Design review of the part built by this model. Coordinates are the model's own, in mm. A direction names the side the tool comes from. Give positions to 0.01 mm unless a question says otherwise; leave off trailing zeros. Loops run counter-clockwise (first coordinate to the right, second up) from the corner with the lowest first, then second, coordinate; pieces in that order, holes last. Notation, with made-up numbers: (60.5, -3.75) - (95.5, -3.75) arc R18 ccw to (95.5, 12.25) - close; hole circle Ø11 at (0.5, -18). An arc over 180 degrees is marked (long way). Write each question's results on one line, items separated by ' | '.
from build123d import *

# Parameters (mm, degrees)
SKETCH1_R           = 2.2
BOSS_EXTRUDE1_DEPTH = 4
FILLET1_R           = 3
SKETCH2_W           = 4.6228
SKETCH2_H           = 4.6228
BOSS_EXTRUDE2_DEPTH = 2
FILLET2_R           = 0.508
FILLET3_R           = 0.508


with BuildPart() as part:
    # Sketch1 → Boss-Extrude1 (new body)
    with BuildSketch(Plane(origin=(0, 0, 0), x_dir=(0, 0, -1), z_dir=(1, 0, 0))):
        Polygon((-4.5, 4.5), (-17.2, 4.5), (-17.2, -4.5), (29.9, -4.5), (29.9, 4.5), (4.5, 43.87), (-4.5, 43.87), align=None)
        with Locations((25.4, 0)):
            Circle(SKETCH1_R, mode=Mode.SUBTRACT)
        with Locations((0, 13.97)):
            Circle(SKETCH1_R, mode=Mode.SUBTRACT)
        with Locations((0, 39.37)):
            Circle(SKETCH1_R, mode=Mode.SUBTRACT)
        with Locations((-12.7, 0)):
            Circle(SKETCH1_R, mode=Mode.SUBTRACT)
        Polygon((4.5, 4.5), (23.949720405, 4.5), (4.5, 34.647066627), align=None, mode=Mode.SUBTRACT)
    extrude(amount=BOSS_EXTRUDE1_DEPTH)

    # Fillet1
    fillet1_edges = [part.edges().sort_by_distance(p)[0] for p in [
        (2, 43.87, 4.5),
        (2, 43.87, -4.5),
        (2, 4.5, -29.9),
        (2, -4.5, -29.9),
        (2, -4.5, 17.2),
        (2, 4.5, 17.2),
        (2, 4.5, 4.5),
        (2, 34.647066627, -4.5),
        (2, 4.5, -4.5),
        (2, 4.5, -23.949720405),
    ]]
    fillet(fillet1_edges, radius=FILLET1_R)

    # Sketch2 → Boss-Extrude2 (add)
    with BuildSketch(Plane(origin=(4, 0, 0), x_dir=(0, 0, -1), z_dir=(1, 0, 0))):
        Rectangle(SKETCH2_W, SKETCH2_H)
        with Locations((12.7, 0)):
            Rectangle(SKETCH2_W, SKETCH2_H)
        with Locations((0, 26.67)):
            Rectangle(SKETCH2_W, SKETCH2_H)
    extrude(amount=BOSS_EXTRUDE2_DEPTH)

    # Fillet2
    fillet2_edges = [part.edges().sort_by_distance(p)[0] for p in [
        (5, 2.3114, 2.3114),
        (5, -2.3114, 2.3114),
        (5, -2.3114, -2.3114),
        (5, 2.3114, -2.3114),
        (5, 2.3114, -10.3886),
        (5, -2.3114, -10.3886),
        (5, -2.3114, -15.0114),
        (5, 2.3114, -15.0114),
        (5, 24.3586, -2.3114),
        (5, 28.9814, -2.3114),
        (5, 28.9814, 2.3114),
        (5, 24.3586, 2.3114),
    ]]
    fillet(fillet2_edges, radius=FILLET2_R)

    # Fillet3
    fillet3_edges = [part.edges().sort_by_distance(p)[0] for p in [
        (6, 2.3114, -12.7),
        (6, 0, -15.0114),
        (6, 0, -10.3886),
        (6, -2.3114, -12.7),
        (6, -2.162610245, -14.862610245),
        (6, -2.162610245, -10.537389755),
        (6, 2.162610245, -10.537389755),
        (6, 2.162610245, -14.862610245),
        (6, 0, -2.3114),
        (6, -2.3114, 0),
        (6, 0, 2.3114),
        (6, 2.3114, 0),
        (6, -2.162610245, 2.162610245),
        (6, 2.162610245, 2.162610245),
        (6, 2.162610245, -2.162610245),
        (6, -2.162610245, -2.162610245),
        (6, 26.67, 2.3114),
        (6, 28.9814, 0),
        (6, 26.67, -2.3114),
        (6, 24.3586, 0),
        (6, 24.507389755, 2.162610245),
        (6, 24.507389755, -2.162610245),
        (6, 28.832610245, -2.162610245),
        (6, 28.832610245, 2.162610245),
    ]]
    fillet(fillet3_edges, radius=FILLET3_R)


solid = part.part
(1) Tool access review of faces 4 (the flat face through (1.97, 17.49, -15.57)), 5 (the flat face through (5, 28.981, 0)), 6 (the flat face through (5, 0, -2.311)), 7 (the flat face through (2, 4.5, 11)): name each direction out of +Z, -Z, +X, -X, +Y, -Y from which nothing blocks a thin tool from reaching the whole face with its end or side.
Answers below:
face 4: +X, -X | face 5: +Z, -Z, +X, +Y | face 6: +X, +Y, -Y | face 7: +Z, +X, -X, +Y
(2) Draft analysis for pull direction Y (two halves, no side actions). For faces 1 (the flat face through (5, 0, 2.311)), 2 (the cylindrical face through (2.03, -3.6, 16.34)), 3 (the flat face through (5, 2.311, 0)), state which applies: pulls with the +Y half, pulls with the -Y half, needs draft (parallel to the pull), parting line crosses it, or undercut.
Answers below:
face 1: needs draft | face 2: pulls with the -Y half | face 3: undercut
(3) Take a section at C-C on x = 2.3. Give the boundary of the cut face in (y, z), plus the area to 3 significant figures.
Answers below:
outline: (-4.5, -26.9) arc R3 ccw to (-1.5, -29.9) - (3.62, -29.9) arc R3 ccw to (5.24, -29.42) - (42.5, -5.39) arc R3 ccw to (43.87, -2.87) - (43.87, 1.5) arc R3 ccw to (40.87, 4.5) - (7.5, 4.5) arc R3 cw to (4.5, 7.5) - (4.5, 14.2) arc R3 ccw to (1.5, 17.2) - (-1.5, 17.2) arc R3 ccw to (-4.5, 14.2) - close; hole circle Ø4.4 at (0, -25.4); hole circle Ø4.4 at (0, 12.7); hole (4.5, -18.44) arc R3 ccw to (9.13, -20.96) - (26.09, -10.02) arc R3 ccw to (24.46, -4.5) - (7.5, -4.5) arc R3 ccw to (4.5, -7.5) - close; hole circle Ø4.4 at (13.97, 0); hole circle Ø4.4 at (39.37, 0) | area: 946 mm2
(4) Insertion check: P1, Ø5, axis at y = 7.5, z = 8.5, coming from the -X side; P2, Ø3, axis at x = 2, z = -10.5, coming from the +Y side (3 decimals); P3, Ø1.2, axis at x = 5, y = -1, coming from the +Z side; P4, Ø1.2, axis at x = 4.5, y = 26, coming from the -Z side. Each pin has a flat end and moves straight along its axis. Give the tip position at first contact, or say it passes through.
Answers below:
P1: through | P2: y = 36.895 | P3: z = 2.31 | P4: z = -16.24
(5) Take a section at D-D on y = 39.37. Give the boundary of the cut face in (x, z), plus the area to 3 significant figures.
Answers below:
outline: (0, -7.4) - (4, -7.4) - (4, -2.2) - (0, -2.2) - close; (0, 2.2) - (4, 2.2) - (4, 4.5) - (0, 4.5) - close | area: 30.0 mm2
(6) Take a section at A-A on z = 12.7. Give the boundary of the cut face in (x, y), plus the area to 3 significant figures.
Answers below:
outline: (0, -4.5) - (4, -4.5) - (4, -2.2) - (0, -2.2) - close; (0, 2.2) - (4, 2.2) - (4, 4.5) - (0, 4.5) - close | area: 18.4 mm2
(7) Take a section at B-B on y = 0. Give the boundary of the cut face in (x, z), plus the area to 3 significant figures.
Answers below:
outline: (0, -29.9) - (4, -29.9) - (4, -27.6) - (0, -27.6) - close; (0, -23.2) - (4, -23.2) - (4, -15.01) - (5.49, -15.01) arc R0.51 ccw to (6, -14.5) - (6, -10.9) arc R0.51 ccw to (5.49, -10.39) - (4, -10.39) - (4, -2.31) - (5.49, -2.31) arc R0.51 ccw to (6, -1.8) - (6, 1.8) arc R0.51 ccw to (5.49, 2.31) - (4, 2.31) - (4, 10.5) - (0, 10.5) - close; (0, 14.9) - (4, 14.9) - (4, 17.2) - (0, 17.2) - close | area: 171 mm2
(8) Wall thickness on line 1 along Y through (x, z) = (3.15, 0); line 2 along Z through (x, y) = (3.15, 0.5); line 3 along Z through (x, y) = (3.45, 15): over which ranges is each line inside the solid? List them lowest first. Write a range as from..to.
Answers below:
line 1: -4.5..11.77, 16.17..37.17, 41.57..43.87 | line 2: -29.9..-27.54, -23.26..10.56, 14.84..17.2 | line 3: -23.13..-17.18, -4.5..-1.94, 1.94..4.5
